```python
from build123d import *

# Parameters (mm, degrees)
F1_DEPTH = 25


with BuildPart() as f1:
    # F0 (on Front) → F1 (new body)
    with BuildSketch(Plane.XZ):
        with BuildLine():
            Line((-0.25, 0.4330127019), (-0.25, 17.4982141946))
            ThreePointArc((-0.25, 17.4982141946), (-17.5, 0), (-0.25, -17.4982141946))
            Line((-0.25, -17.4982141946), (-0.25, -0.4330127019))
            ThreePointArc((-0.25, -0.4330127019), (-0.5, 0), (-0.25, 0.4330127019))
        make_face()
        with BuildLine():
            Line((5.75, 0.4330127019), (5.75, 16.5283846761))
            ThreePointArc((5.75, 16.5283846761), (3.0389376966, 17.2341189991), (0.25, 17.4982141946))
            Line((0.25, 17.4982141946), (0.25, 0.4330127019))
            ThreePointArc((0.25, 0.4330127019), (0.4330127019, 0.25), (0.5, 0))
            ThreePointArc((0.5, 0), (0.4330127019, -0.25), (0.25, -0.4330127019))
            Line((0.25, -0.4330127019), (0.25, -17.4982141946))
            ThreePointArc((0.25, -17.4982141946), (3.0389376966, -17.2341189991), (5.75, -16.5283846761))
            Line((5.75, -16.5283846761), (5.75, -0.4330127019))
            ThreePointArc((5.75, -0.4330127019), (5.5, 0), (5.75, 0.4330127019))
        make_face()
        with BuildLine():
            Line((0.25, 0.4330127019), (0.25, 17.4982141946))
            ThreePointArc((0.25, 17.4982141946), (0, 17.5), (-0.25, 17.4982141946))
            Line((-0.25, 17.4982141946), (-0.25, 0.4330127019))
            ThreePointArc((-0.25, 0.4330127019), (0, 0.5), (0.25, 0.4330127019))
        make_face()
        with BuildLine():
            ThreePointArc((-0.25, -17.4982141946), (0, -17.5), (0.25, -17.4982141946))
            Line((0.25, -17.4982141946), (0.25, -0.4330127019))
            ThreePointArc((0.25, -0.4330127019), (0, -0.5), (-0.25, -0.4330127019))
            Line((-0.25, -0.4330127019), (-0.25, -17.4982141946))
        make_face()
        with BuildLine():
            ThreePointArc((5.75, -16.5283846761), (6.0006939438, -16.439028931), (6.25, -16.3458710383))
            Line((6.25, -16.3458710383), (6.25, -0.4330127019))
            ThreePointArc((6.25, -0.4330127019), (6, -0.5), (5.75, -0.4330127019))
            Line((5.75, -0.4330127019), (5.75, -16.5283846761))
        make_face()
        with BuildLine():
            Line((6.25, 0.4330127019), (6.25, 16.3458710383))
            ThreePointArc((6.25, 16.3458710383), (6.0006939438, 16.439028931), (5.75, 16.5283846761))
            Line((5.75, 16.5283846761), (5.75, 0.4330127019))
            ThreePointArc((5.75, 0.4330127019), (6, 0.5), (6.25, 0.4330127019))
        make_face()
        with BuildLine():
            ThreePointArc((6.25, -16.3458710383), (14.4157032433, -9.9215674165), (17.5, 0))
            ThreePointArc((17.5, 0), (14.4157032433, 9.9215674165), (6.25, 16.3458710383))
            Line((6.25, 16.3458710383), (6.25, 0.4330127019))
            ThreePointArc((6.25, 0.4330127019), (6.4330127019, 0.25), (6.5, 0))
            ThreePointArc((6.5, 0), (6.4330127019, -0.25), (6.25, -0.4330127019))
            Line((6.25, -0.4330127019), (6.25, -16.3458710383))
        make_face()
    extrude(amount=F1_DEPTH)


solid = f1.part
```
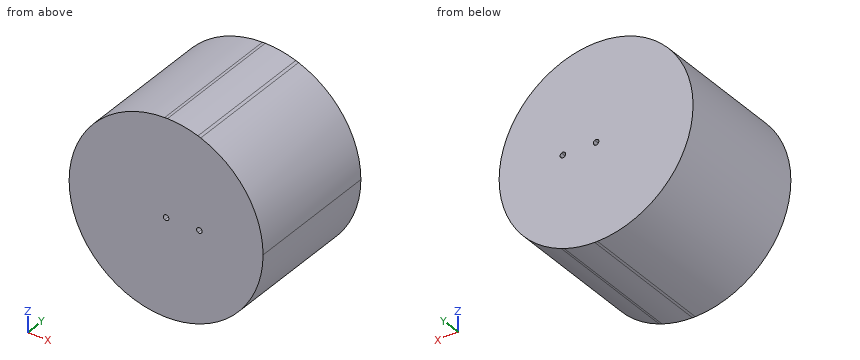
Read the model definition and answer for the solid it produces. Units are mm, in the model's axes. Round coordinates to 2 decimals unless told otherwise and drop trailing zeros. Write each loop counter-clockwise with the first axis right and the second up, starting at its lowest first coordinate (ties: lowest second). Pieces come first, ordered by that corner, then holes. Notation, with made-up numbers: (-21, 2) -> (5, 2) arc R29 cw to (5, 31) -> close; hole circle Ø3 at (70.25, 24). An arc over 180 degrees is marked (long way). Answer in a Markdown table with one row per item. Add a question column.
1) Given P1, Ø1.5, axis at y = -21, z = -9.5, coming from the -X side; P2, Ø6, axis at y = -6, z = 13.5, coming from the -X side; P3, Ø12, axis at y = -4.5, z = -9.5, coming from the +X side, each flat-ended and moving along its own axis, determine where each tip first touches the part or whether it passes through.
2) Find section C-C, the plane x = 5. Determine the outline of the cut face in (y, z), and give its area (3 significant figures).
3) Consider line 1 (X direction, y = -9, z = 7.5); line 2 (Z direction, x = -3, y = -19); line 3 (X direction, y = -11.75, z = 10). Determine where each line is inside the solid, lowest interval first.
4) Find section B-B, the plane z = -8. Determine the outline of the cut face in (x, y).
5) Find section A-A, the plane y = -14.25. Determine the outline of the cut face in (x, z), and give its area (3 significant figures).
Findings below:
| question | item | result |
|---|---|---|
| 1 | P1 | x = -15.16 |
| 1 | P2 | x = -14 |
| 1 | P3 | x = 17.15 |
| 2 | outline | (-25, -16.77) -> (0, -16.77) -> (0, 16.77) -> (-25, 16.77) -> close |
| 2 | area | 839 mm² |
| 3 | line 1 | -15.81 to 15.81 |
| 3 | line 2 | -17.24 to 17.24 |
| 3 | line 3 | -14.36 to 14.36 |
| 4 | outline | (-15.56, -25) -> (15.56, -25) -> (15.56, 0) -> (-15.56, 0) -> close |
| 5 | outline | circle Ø35 at (0, 0); hole circle Ø1 at (0, 0); hole circle Ø1 at (6, 0) |
| 5 | area | 961 mm² |
